Input: part model. Units: mm. Frame: model coordinates. A direction names the side the tool comes from. Give positions to 0.01 mm unless a question says otherwise; leave off trailing zeros. Write each loop counter-clockwise with the first axis right and the second up, starting at its lowest first coordinate (ties: lowest second). Pieces come first, ordered by that corner, then holes. Notation, with made-up numbers: (24, 45) - (47, 45) arc R26 cw to (47, 69) - close; hole circle Ø2 at (45.25, -11). An arc over 180 degrees is marked (long way). Answer as a JSON object with one key per item and string values. Group by question number.
from build123d import *

# Parameters (mm, degrees)
CROQUIS1_W              = 29.5
CROQUIS1_H              = 12.1
SALIENTE_EXTRUIR1_DEPTH = 11.6
CROQUIS2_W              = 29.5
CROQUIS2_H              = 3
SALIENTE_EXTRUIR2_DEPTH = 2.2
CROQUIS3_R              = 0.6
SALIENTE_EXTRUIR3_DEPTH = 3.6


with BuildPart() as part:
    # Croquis1 → Saliente-Extruir1 (new body)
    with BuildSketch(Plane(origin=(0, 0, 0), x_dir=(1, 0, 0), z_dir=(0, 1, 0))):
        Rectangle(CROQUIS1_W, CROQUIS1_H)
    extrude(amount=SALIENTE_EXTRUIR1_DEPTH)

    # Croquis2 → Saliente-Extruir2 (add)
    with BuildSketch(Plane(origin=(0, 11.6, 0), x_dir=(1, 0, 0), z_dir=(0, 1, 0))):
        Rectangle(CROQUIS2_W, CROQUIS2_H)
    extrude(amount=SALIENTE_EXTRUIR2_DEPTH)

    # Croquis3 → Saliente-Extruir3 (add)
    with BuildSketch(Plane.XZ):
        with Locations(Location((-11.5, -1.35, 0), (0, 0, 270))):
            Circle(CROQUIS3_R)
        with Locations(Location((-8, 3.75, 0), (0, 0, 270))):
            Circle(CROQUIS3_R)
        with Locations(Location((-4.5, -1.35, 0), (0, 0, 270))):
            Circle(CROQUIS3_R)
        with Locations(Location((-1, 3.75, 0), (0, 0, 270))):
            Circle(CROQUIS3_R)
        with Locations(Location((2.5, -1.35, 0), (0, 0, 270))):
            Circle(CROQUIS3_R)
        with Locations(Location((6, 3.75, 0), (0, 0, 270))):
            Circle(CROQUIS3_R)
        with Locations(Location((9.5, -1.35, 0), (0, 0, 270))):
            Circle(CROQUIS3_R)
        with Locations(Location((13, 3.75, 0), (0, 0, 270))):
            Circle(CROQUIS3_R)
    extrude(amount=SALIENTE_EXTRUIR3_DEPTH)


solid = part.part
1) Cut plane A-A on y = -0.5. Return the cut outline in (x, z), and give its area (3 significant figures).
2) Pin query (flat end, axial travel): P1, Ø2.5, axis at x = -6.5, z = 4.5, coming from the +Y side; P2, Ø1.8, axis at x = -1.5, y = 13, coming from the +Z side. Return the tip coordinate at first contact, or that it passes through.
3) Cut plane C-C on x = 5. Return the cut outline in (y, z), and give its area (3 significant figures).
4) Line query: line 1 along X through (y, z) = (-2.25, 4); line 2 along Y through (x, z) = (7, -0.25); line 3 along Y through (x, z) = (10.5, 3). Output: solid intervals per line, ascending. Write a range as from..to.
5) Cut plane D-D on z = -0.25. Return the cut outline in (x, y).
6) Mould query, pull axis X, two halves, no side actions, for faces 1 (the face through (-12.03, -1.77, -1.63)), 2 (the face through (14.75, 7, 0)), 3 (the face through (-14.75, 7, 0)), 4 (the face through (9.5, -3.6, -1.3)). Classes: +X half, -X half, draft (parallel to the pull), parting line (faces both ways), or undercut.
7) Reachability of faces 5 (the face through (0, 13, 1.5)), 6 (the face through (12.414, -1.775, 3.88)), 7 (the face through (0, 11.6, -4)) from +Z, -Z, +X, -X, +Y, -Y: full face, straight path, thin tool, end or side. Return the list, or none.
8) Cut plane B-B on z = 3.75. Return the cut outline in (x, y), and give its area (3 significant figures).
Filled in:
{
 "1": {"outline": "circle Ø1.2 at (-11.5, -1.35); circle Ø1.2 at (-8, 3.75); circle Ø1.2 at (-4.5, -1.35); circle Ø1.2 at (-1, 3.75); circle Ø1.2 at (2.5, -1.35); circle Ø1.2 at (6, 3.75); circle Ø1.2 at (9.5, -1.35); circle Ø1.2 at (13, 3.75)", "area": "9.05 mm²"},
 "2": {"P1": "stops at y = 11.6", "P2": "stops at z = 1.5"},
 "3": {"outline": "(0, -6.05) - (11.6, -6.05) - (11.6, -1.5) - (13.8, -1.5) - (13.8, 1.5) - (11.6, 1.5) - (11.6, 6.05) - (0, 6.05) - close", "area": "147 mm²"},
 "4": {"line 1": "x = -8.55..-7.45, -1.55..-0.45, 5.45..6.55, 12.45..13.55", "line 2": "y = 0..13.8", "line 3": "y = 0..11.6"},
 "5": {"outline": "(-14.75, 0) - (14.75, 0) - (14.75, 13.8) - (-14.75, 13.8) - close"},
 "6": {"face 1": "undercut", "face 2": "+X half", "face 3": "-X half", "face 4": "draft"},
 "7": {"face 5": "+Z, +X, -X, +Y", "face 6": "-Y", "face 7": "-Z, +X, -X, +Y"},
 "8": {"outline": "(-14.75, 0) - (-8.6, 0) - (-8.6, -3.6) - (-7.4, -3.6) - (-7.4, 0) - (-1.6, 0) - (-1.6, -3.6) - (-0.4, -3.6) - (-0.4, 0) - (5.4, 0) - (5.4, -3.6) - (6.6, -3.6) - (6.6, 0) - (12.4, 0) - (12.4, -3.6) - (13.6, -3.6) - (13.6, 0) - (14.75, 0) - (14.75, 11.6) - (-14.75, 11.6) - close", "area": "359 mm²"}
}
